Read the model definition and answer for the solid it produces. Units are mm, in the model's axes. Round coordinates to 2 decimals unless told otherwise and drop trailing zeros. Order: outer loops, then holes, each group sorted by start corner. A loop starts at its lowest first (then second) coordinate and runs counter-clockwise, first axis right, second up. Notation, with made-up numbers: (-30, 82) -> (14, 82) arc R26 cw to (14, 105) -> close; hole circle Ø9 at (-39, 29.5). An arc over 180 degrees is marked (long way). One line per item, written item: value. Start each with the question number.
1. The mould has two halves that part along Z. Classify faces 1 (the face through (9.896, 433.581, 4.103)), 2 (the face through (-7.2, 0, 3.9)), 3 (the face through (-7.93, 433.58, -0.35)): released by +Z, released by -Z, zero draft, split by the parting line, or undercut.
2. Consider line 1 (Z direction, x = 0, y = 438); line 2 (X direction, y = 523.5, z = 1.5). Determine where each line is inside the solid, lowest interval first.
3. Section C-C (y = 498) is taken. Give the vertices of the cut face in (x, z) (1 decimal).
4. Section A-A (x = 0) is taken. Give the vertices of the cut face in (y, z), then the cut area to 3 significant figures.
5. Flat-ended cylindrical pins translate along their axes: pin 1 Ø1 at (y, z) = (843.5, -8.5) entering from -X; pin 2 Ø1 at (y, z) = (481, -7) entering from +X; pin 3 Ø3.5 at (y, z) = (844.5, 7.5) entering from +X; pin 4 Ø12 at (y, z) = (172, 2) entering from +X. Find the tip coordinate at first contact, or state that the pin passes through.
6. Section B-B (z = 0) is taken. Give the vertices of the cut face in (x, y) (1 decimal).
from build123d import *

# Parameters (mm, degrees)
SKETCH1_R           = 10.71245
SKETCH1_R_2         = 7.9375
BOSS_EXTRUDE1_DEPTH = 879.475
SKETCH2_W           = 9.144
SKETCH2_H           = 21.4249
CUT_EXTRUDE1_DEPTH  = 108.585


with BuildPart() as part:
    # Sketch1 → Boss-Extrude1 (new body)
    with BuildSketch(Plane(origin=(0, 0, 0), x_dir=(1, 0, 0), z_dir=(0, 1, 0))):
        Circle(SKETCH1_R)
        Circle(SKETCH1_R_2, mode=Mode.SUBTRACT)
    extrude(amount=BOSS_EXTRUDE1_DEPTH)

    # Sketch2 → Cut-Extrude1 (cut)
    with BuildSketch(Plane(origin=(0, 879.475, 0), x_dir=(1, 0, 0), z_dir=(0, 1, 0))):
        Rectangle(SKETCH2_W, SKETCH2_H)
    extrude(amount=-CUT_EXTRUDE1_DEPTH, mode=Mode.SUBTRACT)


solid = part.part
Answer:
1. face 1: split by the parting line
1. face 2: zero draft
1. face 3: undercut
2. line 1: -10.71 to -7.94, 7.94 to 10.71
2. line 2: -10.61 to -7.79, 7.79 to 10.61
3. outline: circle Ø21.4 at (0, 0); hole circle Ø15.9 at (0, 0)
4. outline: (0, -10.71) -> (770.89, -10.71) -> (770.89, -7.94) -> (0, -7.94) -> close; (0, 7.94) -> (770.89, 7.94) -> (770.89, 10.71) -> (0, 10.71) -> close
4. area: 4,280 mm^2
5. pin 1: x = -7.12
5. pin 2: x = 8.52
5. pin 3: x = 9.04
5. pin 4: x = 10.71
6. outline: (-10.7, 0) -> (-7.9, 0) -> (-7.9, 879.5) -> (-10.7, 879.5) -> close; (7.9, 0) -> (10.7, 0) -> (10.7, 879.5) -> (7.9, 879.5) -> close
